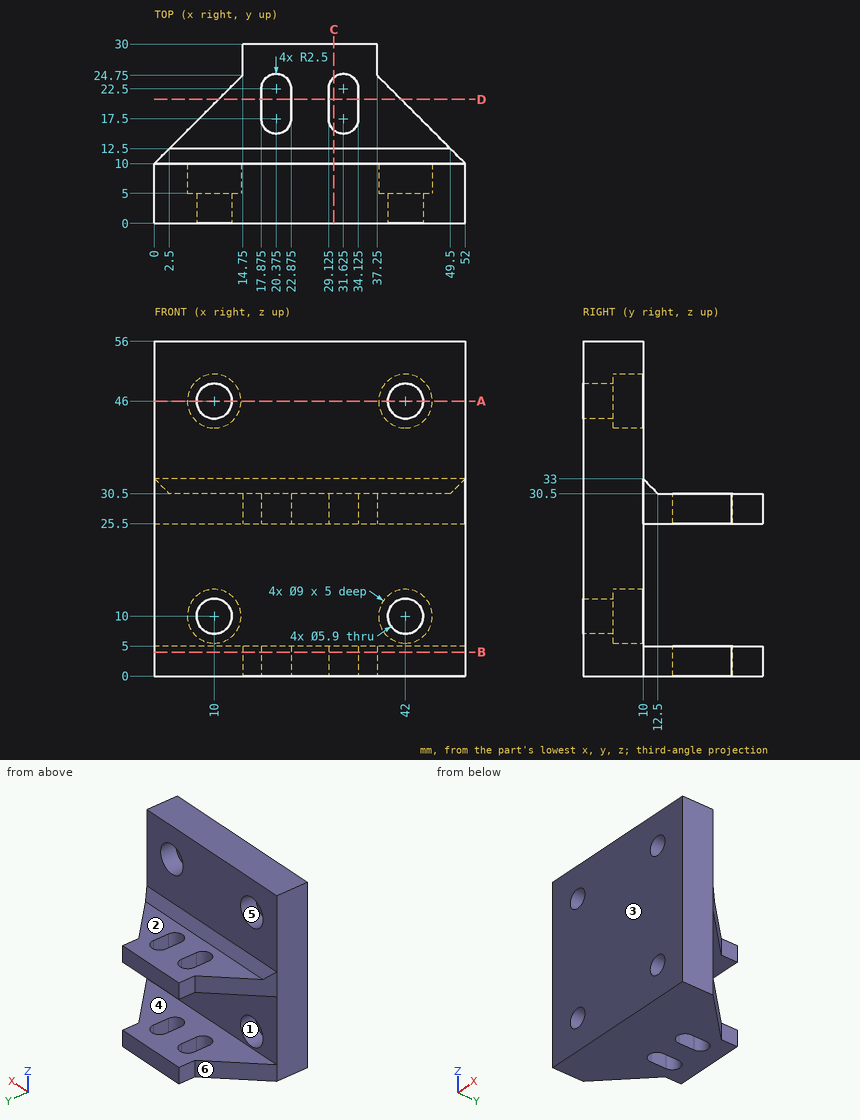
Geometry: see drawing. Coordinates: mm, zero at the bounding-box minimum. A direction names the side the tool comes from. Round coordinates to 2 decimals unless told otherwise and drop trailing zeros. Order: outer loops, then holes, each group sorted by start corner. A loop starts at its lowest first (then second) coordinate and runs counter-clockwise, first axis right, second up. Notation, with made-up numbers: (40, -7.5) - (92, -7.5) arc R29 cw to (92, 28.5) - close; hole circle Ø2 at (-36, 83.25). An arc over 180 degrees is marked (long way). One line per question, with ' | ' between items. Start each with the question number.
1) Ray query, probe 1 along X at (y, z) = (7.4, 46); probe 2 along X at (y, z) = (1.5, 10); probe 3 along Z at (x, y) = (42, 6.6). Return the intervals inside material, ascending.
2) Cut plane C-C, the plane x = 30. Return the cut outline in (y, z), then the cut area to 3 significant figures.
3) Cut plane A-A, the plane z = 46. Return the cut outline in (x, y).
4) Pull-direction query (Z, two-part tool) for the marked faces 1, 2 and 3; classes: +Z half, -Z half, draft (parallel to the pull), parting line (faces both ways), or undercut.
5) Cut plane D-D, the plane y = 20.75. Return the cut outline in (x, z) (3 decimals), then the cut area to 3 significant figures.
6) Contact query for flat-ended pins moving along their axis: P1, Ø5.5, axis at y = 20.5, z = 3, coming from the +X side; P2, Ø10, axis at x = 10, z = 10.5, coming from the +Y side; P3, Ø7, axis at x = 10, z = 46, coming from the +Y side. Output: stop coordinate, or through.
7) Set-up query: the marked faces 4, 5 and 6. Return all of +Z, -Z, +X, -X, +Y, -Y with unobstructed straight access to the full face (end or side cutting, diameter ignored); none if empty.
8) Cut plane B-B, the plane z = 4. Give the number of separate pieces and of enclosed holes in the cut face, then the cut area to 3 significant figures.
Worked out:
1) probe 1: x = 0 to 5.5, 14.5 to 37.5, 46.5 to 52 | probe 2: x = 0 to 7.05, 12.95 to 39.05, 44.95 to 52 | probe 3: z = 0 to 5.5, 14.5 to 41.5, 50.5 to 56
2) outline: (0, 0) - (15.6, 0) - (15.6, 5) - (10, 5) - (10, 25.5) - (15.6, 25.5) - (15.6, 30.5) - (12.5, 30.5) - (10, 33) - (10, 56) - (0, 56) - close; (24.4, 0) - (30, 0) - (30, 5) - (24.4, 5) - close; (24.4, 25.5) - (30, 25.5) - (30, 30.5) - (24.4, 30.5) - close | area: 675 mm^2
3) outline: (0, 0) - (7.05, 0) - (7.05, 5) - (5.5, 5) - (5.5, 10) - (0, 10) - close; (12.95, 0) - (39.05, 0) - (39.05, 5) - (37.5, 5) - (37.5, 10) - (14.5, 10) - (14.5, 5) - (12.95, 5) - close; (44.95, 0) - (52, 0) - (52, 10) - (46.5, 10) - (46.5, 5) - (44.95, 5) - close
4) face 1: undercut | face 2: +Z half | face 3: draft
5) outline: (10.75, 0) - (17.875, 0) - (17.875, 5) - (10.75, 5) - close; (10.75, 25.5) - (17.875, 25.5) - (17.875, 30.5) - (10.75, 30.5) - close; (22.875, 0) - (29.125, 0) - (29.125, 5) - (22.875, 5) - close; (22.875, 25.5) - (29.125, 25.5) - (29.125, 30.5) - (22.875, 30.5) - close; (34.125, 0) - (41.25, 0) - (41.25, 5) - (34.125, 5) - close; (34.125, 25.5) - (41.25, 25.5) - (41.25, 30.5) - (34.125, 30.5) - close | area: 205 mm^2
6) P1: stops at x = 44.25 | P2: stops at y = 10 | P3: stops at y = 5
7) face 4: +X, -X, +Y | face 5: +Y | face 6: +Z, -Z, -X, +Y
8) separate pieces: 1 | enclosed holes: 2 | area: 1,100 mm^2
